Geometry check sheet. Reference: the model listing, model coordinates, mm. A direction names the side the tool comes from. Give positions to 0.01 mm unless a question says otherwise; leave off trailing zeros. Write each loop counter-clockwise with the first axis right and the second up, starting at its lowest first coordinate (ties: lowest second). Pieces come first, ordered by that corner, then holes. Notation, with made-up numbers: (73, 29.5) -> (105, 29.5) arc R12 cw to (105, 36.5) -> close; hole circle Ø1 at (-5.5, -36.75). An arc over 180 degrees is marked (long way). Use a Markdown table: item, result. Add a question column.
Autodesk Inventor part; units mm, degrees
ref_plane "YZ Plane" through (0, 0, 0) normal (1, 0, 0) x (0, 1, 0)
ref_plane "XZ Plane" through (0, 0, 0) normal (0, 1, 0) x (-1, 0, 0)
ref_plane "XY Plane" through (0, 0, 0) normal (0, 0, 1) x (1, 0, 0)
sketch "Sketch1" plane through (0, 0, 0) normal (0, 0, 1) x (1, 0, 0)
  line L0 (-15, -30) -> (15, -30)
  line L1 (15, -30) -> (15, 30)
  line L2 (15, 30) -> (-15, 30)
  line L3 (-15, 30) -> (-15, -30)
  line L4 (-15, -30) -> (15, 30) construction
  line L5 (15, -30) -> (-15, 30) construction
  line L6 (-12, -27) -> (12, -27)
  line L7 (12, -27) -> (12, 27)
  line L8 (12, 27) -> (-12, 27)
  line L9 (-12, 27) -> (-12, -27)
  line L10 (-12, -27) -> (12, 27) construction
  line L11 (12, -27) -> (-12, 27) construction
  point P0 (0, 0)
  dimension "d0" = 30
  dimension "d1" = 60
  dimension "d2" = 24
  dimension "d3" = 54
extrude "Extrusion1" add sketch "Sketch1" along normal blind 200
sketch "Sketch2" plane through (-15, -30, 0) normal (-1, 0, 0) x (0, 0, 1)
  circle A0 centre (188.5, 50) radius 2.75
  circle A1 centre (188.5, 10) radius 2.75
  line L0 (200, 60) -> (200, 0)
  line L1 (0, 0) -> (200, 0)
  line L2 (0, 60) -> (200, 60)
  point P0 (0, 30)
  dimension "d6" = 5.5
  dimension "d7" = 5.5
  dimension "d8" = 11.5
  dimension "d9" = 10
  dimension "d10" = 11.5
  dimension "d11" = 10
extrude "Extrusion2" cut sketch "Sketch2" against normal blind 30
sketch "Sketch3" plane through (-15, 30, 0) normal (0, 1, 0) x (1, 0, 0)
  circle A0 centre (15, -73) radius 2.75
  circle A1 centre (15, -57) radius 2.75
  line L0 (0, 0) -> (0, -200)
  line L1 (30, -200) -> (0, -200)
  circle A2 centre (15, -190) radius 2.75
  line L2 (30, 0) -> (30, -200)
  point P0 (15, 0)
  dimension "d14" = 5.5
  dimension "d15" = 5.5
  dimension "d16" = 15
  dimension "d17" = 15
  dimension "d18" = 127
  dimension "d19" = 16
  dimension "d40" = 5.5
  dimension "d41" = 10
  dimension "d42" = 15
extrude "Extrusion3" cut sketch "Sketch3" against normal blind 60
sketch "Sketch4" plane through (-15, -30, 0) normal (-1, 0, 0) x (0, 0, 1)
  circle A0 centre (150, 30) radius 20
  line L0 (125, 50) -> (175, 50)
  line L1 (175, 50) -> (175, 10)
  line L2 (175, 10) -> (125, 10)
  line L3 (125, 10) -> (125, 50)
  line L4 (125, 50) -> (175, 10) construction
  line L5 (175, 50) -> (125, 10) construction
  circle A1 centre (175, 50) radius 2.75
  circle A2 centre (175, 10) radius 2.75
  circle A3 centre (125, 10) radius 2.75
  circle A4 centre (125, 50) radius 2.75
  line L6 (200, 60) -> (200, 0)
  line L7 (0, 0) -> (200, 0)
  circle A5 centre (75, 50) radius 2.75
  circle A6 centre (100, 30) radius 20
  circle A7 centre (125, 50) radius 2.75
  circle A8 centre (125, 10) radius 2.75
  circle A9 centre (75, 10) radius 2.75
  circle A10 centre (25, 50) radius 2.75
  circle A11 centre (50, 30) radius 20
  circle A12 centre (75, 50) radius 2.75
  circle A13 centre (75, 10) radius 2.75
  circle A14 centre (25, 10) radius 2.75
  circle A15 centre (-25, 50) radius 2.75
  circle A16 centre (0, 30) radius 20
  circle A17 centre (25, 50) radius 2.75
  circle A18 centre (25, 10) radius 2.75
  circle A19 centre (-25, 10) radius 2.75
  circle A20 centre (-75, 50) radius 2.75
  circle A21 centre (-50, 30) radius 20
  circle A22 centre (-25, 50) radius 2.75
  circle A23 centre (-25, 10) radius 2.75
  circle A24 centre (-75, 10) radius 2.75
  circle A25 centre (-125, 50) radius 2.75
  circle A26 centre (-100, 30) radius 20
  circle A27 centre (-75, 50) radius 2.75
  circle A28 centre (-75, 10) radius 2.75
  circle A29 centre (-125, 10) radius 2.75
  circle A30 centre (-175, 50) radius 2.75
  circle A31 centre (-150, 30) radius 20
  circle A32 centre (-125, 50) radius 2.75
  circle A33 centre (-125, 10) radius 2.75
  circle A34 centre (-175, 10) radius 2.75
  circle A35 centre (-225, 50) radius 2.75
  circle A36 centre (-200, 30) radius 20
  circle A37 centre (-175, 50) radius 2.75
  circle A38 centre (-175, 10) radius 2.75
  circle A39 centre (-225, 10) radius 2.75
  circle A40 centre (-275, 50) radius 2.75
  circle A41 centre (-250, 30) radius 20
  circle A42 centre (-225, 50) radius 2.75
  circle A43 centre (-225, 10) radius 2.75
  circle A44 centre (-275, 10) radius 2.75
  circle A45 centre (-325, 50) radius 2.75
  circle A46 centre (-300, 30) radius 20
  circle A47 centre (-275, 50) radius 2.75
  circle A48 centre (-275, 10) radius 2.75
  circle A49 centre (-325, 10) radius 2.75
  point P0 (0, 30)
  dimension "d22" = 40
  dimension "d23" = 50
  dimension "d24" = 40
  dimension "d25" = 5.5
  dimension "d26" = 5.5
  dimension "d27" = 5.5
  dimension "d28" = 5.5
  dimension "d29" = 50
  dimension "d30" = 10
  dimension "d33" = 50
extrude "Extrusion4" cut sketch "Sketch4" against normal blind 60 contours A0 | A4 L3 L0 | L0 L3 A4 | A1 L1 L0 | L0 L1 A1 | A2 L1 L2 | L2 L1 A2 | A3 L3 L2 | L2 L3 A3
sketch "Sketch5" plane through (-15, -30, 0) normal (-1, 0, 0) x (0, 0, 1)
  circle A0 centre (38.5, 50) radius 2.75
  circle A1 centre (91.5, 50) radius 2.75
  circle A2 centre (91.5, 10) radius 2.75
  circle A3 centre (38.5, 10) radius 2.75
  line L0 (0, 60) -> (200, 60)
  line L1 (0, 60) -> (0, 0)
  point P0 (0, 30)
  dimension "d43" = 5.5
  dimension "d44" = 5.5
  dimension "d45" = 5.5
  dimension "d46" = 5.5
  dimension "d47" = 40
  dimension "d48" = 40
  dimension "d49" = 40
  dimension "d50" = 53
  dimension "d51" = 53
  dimension "d52" = 10
  dimension "d53" = 53
  dimension "d54" = 38.5
extrude "Extrusion5" cut sketch "Sketch5" against normal blind 60
properties part number "SupportExtrusion" material "Aluminum 6061"
1) Sectioned sample at D-D, the plane y = -5. Enter the section's corners in (x, z), and give its area (3 significant figures).
2) Material ranges on probe 1 along Y at (x, z) = (-14.05, 91.5); probe 2 along X at (y, z) = (-20.5, 179); probe 3 along Y at (x, z) = (6, 45), recorded low to high. Write a range as [from, to].
3) Gauge pin test, flat end, axial feed: P1, Ø12, axis at x = -0.5, y = -6.5, coming from the +Z side. Record the tip position at first contact, or that the pin passes through.
4) Sectioned sample at A-A, the plane z = 57. Enter the section's corners in (x, y), and give its area (3 significant figures).
5) Tool access check on faces 1 (the face through (0, -27, 99)), 2 (the face through (13.479, -19.879, 88.753)). Record the directions out of +Z, -Z, +X, -X, +Y, -Y that give a thin tool (end or side, any length) a straight path to the whole face; none if there is none.
6) Sectioned sample at C-C, the plane z = 125. Enter the section's corners in (x, y), and give its area (3 significant figures).
7) Draft check along Z on faces 3 (the face through (15, 0, 99)), 4 (the face through (-12.3, 2.4, 0)), 5 (the face through (-13.521, 20.121, 88.753)). Enter one of: +Z half, -Z half, draft (parallel to the pull), parting line (faces both ways), or undercut.
8) Sectioned sample at B-B, the plane x = -10.25. Enter the section's corners in (y, z), and give its area (3 significant figures).
Check values:
| question | item | result |
|---|---|---|
| 1 | outline | (-15, 0) -> (-12, 0) -> (-12, 130.64) -> (-15, 130.64) -> close; (-15, 169.36) -> (-12, 169.36) -> (-12, 200) -> (-15, 200) -> close; (12, 0) -> (15, 0) -> (15, 130.64) -> (12, 130.64) -> close; (12, 169.36) -> (15, 169.36) -> (15, 200) -> (12, 200) -> close |
| 1 | area | 968 mm² |
| 2 | probe 1 | [-30, -22.75], [-17.25, 17.25], [22.75, 30] |
| 2 | probe 2 | [-15, -12], [12, 15] |
| 2 | probe 3 | [-30, -27], [27, 30] |
| 3 | P1 | through |
| 4 | outline | (-15, -30) -> (-2.75, -30) -> (-2.75, -27) -> (-12, -27) -> (-12, 27) -> (-2.75, 27) -> (-2.75, 30) -> (-15, 30) -> close; (2.75, -30) -> (15, -30) -> (15, 30) -> (2.75, 30) -> (2.75, 27) -> (12, 27) -> (12, -27) -> (2.75, -27) -> close |
| 4 | area | 471 mm² |
| 5 | face 1 | +Z, -Z |
| 5 | face 2 | +X, -X |
| 6 | outline | (-15, -30) -> (15, -30) -> (15, -22.75) -> (12, -22.75) -> (12, -27) -> (-12, -27) -> (-12, -22.75) -> (-15, -22.75) -> close; (-15, -17.25) -> (-12, -17.25) -> (-12, 17.25) -> (-15, 17.25) -> close; (-15, 22.75) -> (-12, 22.75) -> (-12, 27) -> (12, 27) -> (12, 22.75) -> (15, 22.75) -> (15, 30) -> (-15, 30) -> close; (12, -17.25) -> (15, -17.25) -> (15, 17.25) -> (12, 17.25) -> close |
| 6 | area | 438 mm² |
| 7 | face 3 | draft |
| 7 | face 4 | -Z half |
| 7 | face 5 | undercut |
| 8 | outline | (-30, 0) -> (-27, 0) -> (-27, 200) -> (-30, 200) -> close; (27, 0) -> (30, 0) -> (30, 200) -> (27, 200) -> close |
| 8 | area | 1,200 mm² |
